from build123d import *

# Parameters (mm, degrees)
F0_W     = 50.8
F0_H     = 50.8
F0_W_2   = 44.45
F0_H_2   = 44.45
F1_DEPTH = 495.3
F3_D     = 12.7
F3_DEPTH = 12.7
F3_TIP   = 3.8154649308
F5_D     = 12.7
F5_DEPTH = 12.7
F5_TIP   = 3.8154649308


# Not quite as in the source:
# - a length typed as a fraction of an inch, garbled in the dataset ("3 / 203.2 mm" for 3/8 in), is restored


with BuildPart() as f1:
    # F0 (on Front) → F1 (new body, symmetric)
    with BuildSketch(Plane.XZ):
        Rectangle(F0_W, F0_H)
        Rectangle(F0_W_2, F0_H_2, mode=Mode.SUBTRACT)
    extrude(amount=F1_DEPTH, both=True)

    # F3
    with Locations(Plane.XY.offset(25.4)):
        with Locations((0, 63.5), (0, -63.5)):
            Hole(F3_D / 2, depth=F3_DEPTH)
            with Locations((0, 0, -(F3_DEPTH + F3_TIP / 2))):  # 118° drill point
                Cone(0, F3_D / 2, F3_TIP, mode=Mode.SUBTRACT)

    # F5
    with Locations(Plane.YZ.offset(25.4)):
        with Locations((44.45, 0), (-44.45, 0)):
            Hole(F5_D / 2, depth=F5_DEPTH)
            with Locations((0, 0, -(F5_DEPTH + F5_TIP / 2))):  # 118° drill point
                Cone(0, F5_D / 2, F5_TIP, mode=Mode.SUBTRACT)


solid = f1.part
Work out the finished part from the listing and answer in its coordinate system (mm). A direction names the side the tool comes from. Round coordinates to 2 decimals unless told otherwise and drop trailing zeros. Order: outer loops, then holes, each group sorted by start corner. A loop starts at its lowest first (then second) coordinate and runs counter-clockwise, first axis right, second up. Notation, with made-up numbers: M 46.25,45.5 L 102.25,45.5 A12 ccw 102.25,67.5 Z; hole C 21,50 d1. An arc over 180 degrees is marked long. Put each result on its own line as item: value. Start each with the question number.
Q1. Section A-A, the plane y = -372 is taken. Write down the section's boundary in (x, z) (3 decimals), and give its area (3 significant figures).
Q2. A tool of negligible diameter and unlimited length cuts with its end or side. For faces 1 (the flat face through (25.4, -7, 0)), 2 (the flat face through (-22.225, -7, 0)), from which of +Z, -Z, +X, -X, +Y, -Y can it reach the whole face along a straight path? Write none if from no direction.
Q3. For a pull along Z with two mould halves and no side action, classify faces 3 (the flat face through (0, -7, 22.225)), 4 (the flat face through (0, -7, 25.4)), 5 (the flat face through (0, -7, -25.4)) as pulls with the +Z half, pulls with the -Z half, needs draft (parallel to the pull), parting line crosses it, or undercut.
Q4. Straight lines are drawn through the part: L1, parallel to Z at x = -17, y = -101.5 (3 decimals); L2, parallel to X at y = 63, z = 23. For each, find the intervals that lie inside material, in ascending order. Write a range as [from, to].
Q5. Flat-ended cylindrical pins translate along their axes: pin 1 (10 mm diameter, centred on y = -44.45, z = 0, fed in from +X) (3 decimals); pin 2 (5 mm diameter, centred on x = -20, z = -13.5, fed in from +Y). Find the tip coordinate at first contact, or state that the pin passes through.
Findings below:
1. outline: M -25.4,-25.4 L 25.4,-25.4 L 25.4,25.4 L -25.4,25.4 Z; hole M -22.225,-22.225 L 22.225,-22.225 L 22.225,22.225 L -22.225,22.225 Z
1. area: 605 mm^2
2. face 1: +Z, -Z, +X, +Y, -Y
2. face 2: +Y, -Y
3. face 3: undercut
3. face 4: pulls with the +Z half
3. face 5: pulls with the -Z half
4. L1: z = [-25.4, -22.225], [22.225, 25.4]
4. L2: x = [-25.4, -6.33], [6.33, 25.4]
5. pin 1: stops at x = -22.225
5. pin 2: stops at y = 495.3
